```python
from build123d import *

# Parameters (mm, degrees)
ESQUISSE1_R             = 1.1
ESQUISSE1_R_2           = 1.5
ESQUISSE1_W             = 17
ESQUISSE1_H             = 25
BOSS_EXTRU_1_DEPTH      = 2
CONG_1_R                = 2
ENL_V_MAT_EXTRU_1_DEPTH = 2
CONG_2_R                = 4


with BuildPart() as part:
    # Esquisse1 → Boss.-Extru.1 (new body)
    with BuildSketch(Plane.XY):
        with BuildLine():
            Line((9.5, 0), (-9.5, 0))
            Line((-9.5, 0), (-9.5, 80.160865618))
            ThreePointArc((-9.5, 80.160865618), (0, 134.5), (9.5, 80.160865618))
            Line((9.5, 80.160865618), (9.5, 0))
        make_face()
        with Locations((-10.5, 123)):
            Circle(ESQUISSE1_R, mode=Mode.SUBTRACT)
        with Locations((-10.5, 110.5)):
            Circle(ESQUISSE1_R, mode=Mode.SUBTRACT)
        with Locations((10.5, 110.5)):
            Circle(ESQUISSE1_R, mode=Mode.SUBTRACT)
        with Locations((10.5, 123)):
            Circle(ESQUISSE1_R, mode=Mode.SUBTRACT)
        with Locations((0, 132)):
            Circle(ESQUISSE1_R_2, mode=Mode.SUBTRACT)
        with Locations((18.03122292, 124.53122292)):
            Circle(ESQUISSE1_R_2, mode=Mode.SUBTRACT)
        with Locations((25.5, 106.5)):
            Circle(ESQUISSE1_R_2, mode=Mode.SUBTRACT)
        with Locations((18.03122292, 88.46877708)):
            Circle(ESQUISSE1_R_2, mode=Mode.SUBTRACT)
        with Locations((0, 81)):
            Circle(ESQUISSE1_R_2, mode=Mode.SUBTRACT)
        with Locations((-18.03122292, 88.46877708)):
            Circle(ESQUISSE1_R_2, mode=Mode.SUBTRACT)
        with Locations((-25.5, 106.5)):
            Circle(ESQUISSE1_R_2, mode=Mode.SUBTRACT)
        with Locations((-18.03122292, 124.53122292)):
            Circle(ESQUISSE1_R_2, mode=Mode.SUBTRACT)
        with Locations((0, 112.5)):
            Rectangle(ESQUISSE1_W, ESQUISSE1_H, mode=Mode.SUBTRACT)
    extrude(amount=BOSS_EXTRU_1_DEPTH)

    # Congé1
    cong_1_edges = [part.edges().sort_by_distance(p)[0] for p in [
        (-8.5, 125, 1),
        (-8.5, 100, 1),
        (8.5, 100, 1),
        (8.5, 125, 1),
    ]]
    fillet(cong_1_edges, radius=CONG_1_R)

    # Esquisse2 → Enlèv. mat.-Extru.1 (cut)
    with BuildSketch(Plane.XY.offset(2)):
        with BuildLine():
            Line((4.5, 72), (4.5, 50))
            ThreePointArc((4.5, 50), (0, 45.5), (-4.5, 50))
            Line((-4.5, 50), (-4.5, 72))
            ThreePointArc((-4.5, 72), (0, 76.5), (4.5, 72))
        make_face()
        with BuildLine():
            Line((1.5, 41), (1.5, 5))
            ThreePointArc((1.5, 5), (0, 3.5), (-1.5, 5))
            Line((-1.5, 5), (-1.5, 41))
            ThreePointArc((-1.5, 41), (0, 42.5), (1.5, 41))
        make_face()
    extrude(amount=-ENL_V_MAT_EXTRU_1_DEPTH, mode=Mode.SUBTRACT)

    # Congé2
    cong_2_edges = [part.edges().sort_by_distance(p)[0] for p in [
        (9.5, 0, 1),
        (-9.5, 0, 1),
    ]]
    fillet(cong_2_edges, radius=CONG_2_R)


solid = part.part
```
Model file for the job. Use its own axes, mm. A direction names the side the tool comes from. Coordinates: 2 decimals unless noted, no trailing zeros. Order: outer loops, then holes, each group sorted by start corner. A loop starts at its lowest first (then second) coordinate and runs counter-clockwise, first axis right, second up. Notation, with made-up numbers: (10.25, -13.75) -> (65.25, -13.75) arc R27 cw to (65.25, 24.25) -> close; hole circle Ø4 at (-2, -21.75). An arc over 180 degrees is marked (long way). Answer as a JSON object with one key per item and string values. Group by question number.
1) Drill centre lines: L1, parallel to Y at x = 0, z = 1.05; L2, parallel to X at y = 27, z = 0.65; L3, parallel to X at y = 72, z = 0.75. Where is each one in solid material? Low to high.
2) Flat gauge pins, fed straight in: pin 1 (5 mm diameter, centred on x = 25.5, y = 106.5, fed in from +Z); pin 2 (1 mm diameter, centred on x = 2, z = 1, fed in from +Y); pin 3 (0.6 mm diameter, centred on y = 58, z = 0.5, fed in from +X); pin 4 (0.6 mm diameter, centred on y = 24.5, z = 1, fed in from -X). Where does each tip first touch, or does it go through?
3) Cut at B-B, the plane x = -25.5. Write the cut outline in (y, z), then the cut area to 3 significant figures.
4) Cut at A-A, the plane y = 39.5. Write the cut outline in (x, z), then the cut area to 3 significant figures.
5) Pull direction Y, two halves, no side cores. Call faces 3 (the face through (0, 83, 2)), 4 (the face through (-8.297, 1.141, 1.014)), 5 (the face through (-10.738, 121.926, 0.986)): +Y half, -Y half, draft (parallel to the pull), parting line (faces both ways), or undercut.
6) Cut at C-C, the plane y = 106.5. Write the cut outline in (x, z), then the cut area to 3 significant figures.
7) Cut at D-D, the plane z = 1.25. Count the separate pieces of the cut face and the enclosed holes in it, then the cut area to 3 significant figures.
8) Which spindle directions (+Z, -Z, +X, -X, +Y, -Y) get a long thin tool onto all of the face, cutting with end or side? Do faces 1 (the face through (8.297, 1.141, 1.014)), 2 (the face through (0.1, 45.5, 1)). Say none if no direction does.
Check values:
{
 "1": {"L1": "y = 0 to 3.5, 42.5 to 45.5, 76.5 to 79.5, 82.5 to 100, 125 to 130.5, 133.5 to 134.5", "L2": "x = -9.5 to -1.5, 1.5 to 9.5", "L3": "x = -9.5 to -4.5, 4.5 to 9.5"},
 "2": {"pin 1": "stops at z = 2", "pin 2": "stops at y = 134.46", "pin 3": "stops at x = 9.5", "pin 4": "stops at x = -9.5"},
 "3": {"outline": "(94.93, 0) -> (105, 0) -> (105, 2) -> (94.93, 2) -> close; (108, 0) -> (118.07, 0) -> (118.07, 2) -> (108, 2) -> close", "area": "40.3 mm²"},
 "4": {"outline": "(-9.5, 0) -> (-1.5, 0) -> (-1.5, 2) -> (-9.5, 2) -> close; (1.5, 0) -> (9.5, 0) -> (9.5, 2) -> (1.5, 2) -> close", "area": "32.0 mm²"},
 "5": {"face 3": "draft", "face 4": "-Y half", "face 5": "undercut"},
 "6": {"outline": "(-28, 0) -> (-27, 0) -> (-27, 2) -> (-28, 2) -> close; (-24, 0) -> (-8.5, 0) -> (-8.5, 2) -> (-24, 2) -> close; (8.5, 0) -> (24, 0) -> (24, 2) -> (8.5, 2) -> close; (27, 0) -> (28, 0) -> (28, 2) -> (27, 2) -> close", "area": "66.0 mm²"},
 "7": {"separate pieces": "1", "enclosed holes": "15", "area": "3,090 mm²"},
 "8": {"face 1": "+Z, -Z, +X, -Y", "face 2": "+Z, -Z"}
}
